Source: CAD feature listing. Evaluate the final solid. Frame: model axes, mm. Give positions to 0.01 mm unless a question says otherwise; leave off trailing zeros. Order: outer loops, then holes, each group sorted by start corner. A loop starts at its lowest first (then second) coordinate and runs counter-clockwise, first axis right, second up.
1) Section D-D, the plane y = -3.25. Return loops of the section in (x, z).
2) Material intervals for line 1 (Y direction, x = 1, z = 2.4); line 2 (X direction, y = 10, z = 0.75); line 3 (Y direction, x = -18, z = 1), sorted ascending.
3) Section B-B, the plane x = -18. Return loops of the section in (y, z).
4) First-contact query: P1, Ø12, axis at x = 3.5, y = 4, coming from the -Z side. Flat tip, straight axial feed; report the tip coordinate or a pass-through.
5) Section C-C, the plane z = 2.5. Return loops of the section in (x, y), plus the area to 3 significant figures.
6) Section A-A, the plane y = -8. Return loops of the section in (x, z), plus the area to 3 significant figures.
```python
from build123d import *

# Parameters (mm, degrees)
SKETCH_W  = 48
SKETCH_H  = 45.5
SKETCH_R  = 2
PAD_DEPTH = 3
FILLET_R  = 2


with BuildPart() as part:
    # Sketch → Pad (new body)
    with BuildSketch(Plane.XY):
        with Locations((0, -3)):
            Rectangle(SKETCH_W, SKETCH_H)
        with Locations((-18, -3.25)):
            Circle(SKETCH_R, mode=Mode.SUBTRACT)
        with Locations((18, -3.25)):
            Circle(SKETCH_R, mode=Mode.SUBTRACT)
        Polygon((-14, 12.75), (14, 12.75), (14, -12.75), (8.25, -18.75), (-8.25, -18.75), (-14, -12.75), align=None, mode=Mode.SUBTRACT)
    extrude(amount=PAD_DEPTH)

    # Fillet
    fillet_edges = [part.edges().sort_by_distance(p)[0] for p in [
        (-24, -25.75, 1.5),
        (24, -25.75, 1.5),
        (24, 19.75, 1.5),
        (-24, 19.75, 1.5),
    ]]
    fillet(fillet_edges, radius=FILLET_R)


solid = part.part
```
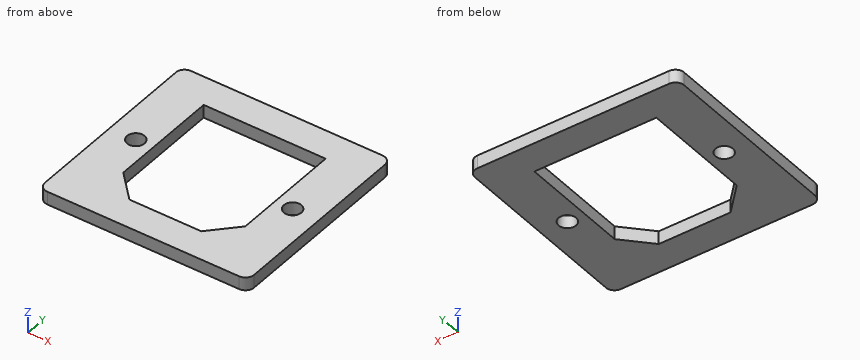
From the geometry:
1. outline: (-24, 0) - (-20, 0) - (-20, 3) - (-24, 3) - close; (-16, 0) - (-14, 0) - (-14, 3) - (-16, 3) - close; (14, 0) - (16, 0) - (16, 3) - (14, 3) - close; (20, 0) - (24, 0) - (24, 3) - (20, 3) - close
2. line 1: y = -25.75 to -18.75, 12.75 to 19.75
2. line 2: x = -24 to -14, 14 to 24
2. line 3: y = -25.75 to -5.25, -1.25 to 19.75
3. outline: (-25.75, 0) - (-5.25, 0) - (-5.25, 3) - (-25.75, 3) - close; (-1.25, 0) - (19.75, 0) - (19.75, 3) - (-1.25, 3) - close
4. P1: passes through
5. outline: (-24, -23.75) arc R2 ccw to (-22, -25.75) - (22, -25.75) arc R2 ccw to (24, -23.75) - (24, 17.75) arc R2 ccw to (22, 19.75) - (-22, 19.75) arc R2 ccw to (-24, 17.75) - close; hole circle Ø4 at (-18, -3.25); hole (-14, -12.75) - (-8.25, -18.75) - (8.25, -18.75) - (14, -12.75) - (14, 12.75) - (-14, 12.75) - close; hole circle Ø4 at (18, -3.25)
5. area: 1,310 mm2
6. outline: (-24, 0) - (-14, 0) - (-14, 3) - (-24, 3) - close; (14, 0) - (24, 0) - (24, 3) - (14, 3) - close
6. area: 60.0 mm2
